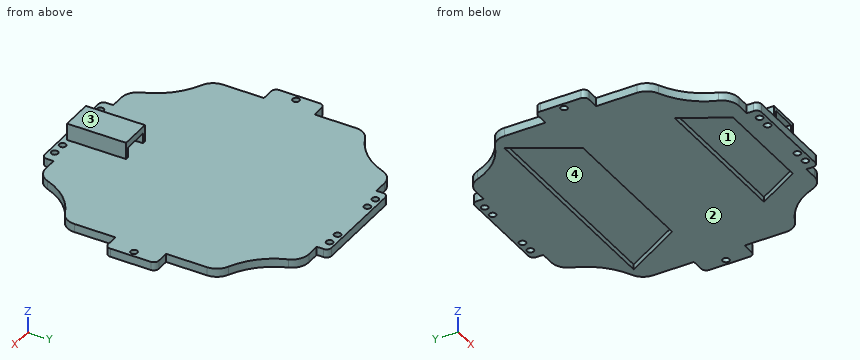
```python
from build123d import *

# Parameters (mm, degrees)
BOSS_EXTRUDE1_DEPTH = 5
SKETCH2_R           = 2
CUT_EXTRUDE1_DEPTH  = 5
CUT_EXTRUDE2_DEPTH  = 3
SKETCH4_W           = 19
SKETCH4_H           = 35
BOSS_EXTRUDE2_DEPTH = 10
SKETCH6_W           = 15
SKETCH6_H           = 8
CUT_EXTRUDE4_DEPTH  = 33
SKETCH7_W           = 15
SKETCH7_H           = 6
CUT_EXTRUDE5_DEPTH  = 2


with BuildPart() as part:
    # Sketch1 → Boss-Extrude1 (new body)
    with BuildSketch(Plane.XY):
        with BuildLine():
            Line((82, 15), (74.70882917, 15))
            Line((74.70882917, 15), (74.70882917, 39.302424721))
            ThreePointArc((74.70882917, 39.302424721), (73.092812163, 44.753005348), (68.767063336, 48.441939777))
            ThreePointArc((68.767063336, 48.441939777), (55.730177295, 57.736884279), (47.382982574, 71.4))
            ThreePointArc((47.382982574, 71.4), (43.723290865, 76.185352772), (37.978728218, 78))
            Line((37.978728218, 78), (30, 78))
            Line((30, 78), (30, 82))
            ThreePointArc((30, 82), (29.121320344, 84.121320344), (27, 85))
            Line((27, 85), (-27, 85))
            ThreePointArc((-27, 85), (-29.121320344, 84.121320344), (-30, 82))
            Line((-30, 82), (-30, 78))
            Line((-30, 78), (-37.978728218, 78))
            ThreePointArc((-37.978728218, 78), (-43.723290865, 76.185352772), (-47.382982574, 71.4))
            ThreePointArc((-47.382982574, 71.4), (-55.730177295, 57.736884279), (-68.767063336, 48.441939777))
            ThreePointArc((-68.767063336, 48.441939777), (-73.092812163, 44.753005348), (-74.70882917, 39.302424721))
            Line((-74.70882917, 39.302424721), (-74.70882917, 15))
            Line((-74.70882917, 15), (-82, 15))
            ThreePointArc((-82, 15), (-84.121320344, 14.121320344), (-85, 12))
            Line((-85, 12), (-85, -12))
            ThreePointArc((-85, -12), (-84.121320344, -14.121320344), (-82, -15))
            Line((-82, -15), (-74.70882917, -15))
            Line((-74.70882917, -15), (-74.70882917, -39.302424721))
            ThreePointArc((-74.70882917, -39.302424721), (-73.092812163, -44.753005348), (-68.767063336, -48.441939777))
            ThreePointArc((-68.767063336, -48.441939777), (-55.730177295, -57.736884279), (-47.382982574, -71.4))
            ThreePointArc((-47.382982574, -71.4), (-43.723290865, -76.185352772), (-37.978728218, -78))
            Line((-37.978728218, -78), (-30, -78))
            Line((-30, -78), (-30, -82))
            ThreePointArc((-30, -82), (-29.121320344, -84.121320344), (-27, -85))
            Line((-27, -85), (27, -85))
            ThreePointArc((27, -85), (29.121320344, -84.121320344), (30, -82))
            Line((30, -82), (30, -78))
            Line((30, -78), (37.978728218, -78))
            ThreePointArc((37.978728218, -78), (43.723290865, -76.185352772), (47.382982574, -71.4))
            ThreePointArc((47.382982574, -71.4), (55.730177295, -57.736884279), (68.767063336, -48.441939777))
            ThreePointArc((68.767063336, -48.441939777), (73.092812163, -44.753005348), (74.70882917, -39.302424721))
            Line((74.70882917, -39.302424721), (74.70882917, -15))
            Line((74.70882917, -15), (82, -15))
            ThreePointArc((82, -15), (84.121320344, -14.121320344), (85, -12))
            Line((85, -12), (85, 12))
            ThreePointArc((85, 12), (84.121320344, 14.121320344), (82, 15))
        make_face()
    extrude(amount=BOSS_EXTRUDE1_DEPTH)

    # Sketch2 → Cut-Extrude1 (cut)
    with BuildSketch(Plane(origin=(0, 0, 0), x_dir=(-1, 0, 0), z_dir=(0, 0, -1))):
        with Locations((81.5, 0)):
            Circle(SKETCH2_R)
        with Locations(Location((-81.5, 0, 0), (0, 0, 180))):
            Circle(SKETCH2_R)
        with Locations((-23, 81.5)):
            Circle(SKETCH2_R)
        with Locations((15, 81.5)):
            Circle(SKETCH2_R)
        with Locations((23, 81.5)):
            Circle(SKETCH2_R)
        with Locations((-15, 81.5)):
            Circle(SKETCH2_R)
        with Locations(Location((-23, -81.5, 0), (0, 0, 180))):
            Circle(SKETCH2_R)
        with Locations(Location((-15, -81.5, 0), (0, 0, 180))):
            Circle(SKETCH2_R)
        with Locations(Location((15, -81.5, 0), (0, 0, 180))):
            Circle(SKETCH2_R)
        with Locations(Location((23, -81.5, 0), (0, 0, 180))):
            Circle(SKETCH2_R)
    extrude(amount=-CUT_EXTRUDE1_DEPTH, mode=Mode.SUBTRACT)

    # Sketch3 → Cut-Extrude2 (cut)
    with BuildSketch(Plane(origin=(0, 0, 0), x_dir=(-1, 0, 0), z_dir=(0, 0, -1))):
        Polygon((-30, -70), (-45, -44.019237886), (45, -44.019237886), (30, -70), align=None)
        Polygon((65, 45), (-65, 45), (-45, 10.358983849), (45, 10.358983849), align=None)
    extrude(amount=-CUT_EXTRUDE2_DEPTH, mode=Mode.SUBTRACT)

    # Sketch4 → Boss-Extrude2 (add)
    with BuildSketch(Plane.XY.offset(5)):
        with Locations((0.2, -64.5)):
            Rectangle(SKETCH4_W, SKETCH4_H)
    extrude(amount=BOSS_EXTRUDE2_DEPTH)

    # Sketch6 → Cut-Extrude4 (cut)
    with BuildSketch(Plane.XZ.offset(82)):
        with Locations((0.2, 9)):
            Rectangle(SKETCH6_W, SKETCH6_H)
    extrude(amount=-CUT_EXTRUDE4_DEPTH, mode=Mode.SUBTRACT)

    # Sketch7 → Cut-Extrude5 (cut)
    with BuildSketch(Plane(origin=(0, -47, 0), x_dir=(1, 0, 0), z_dir=(0, 1, 0))):
        with Locations((0.2, -8)):
            Rectangle(SKETCH7_W, SKETCH7_H)
    extrude(amount=-CUT_EXTRUDE5_DEPTH, mode=Mode.SUBTRACT)


solid = part.part
```
Part model, mm, in its own coordinate system. Face numbers are marked on the shaded views. A direction names the side the tool comes from. Coordinates: 2 decimals unless noted, no trailing zeros. Write each loop counter-clockwise with the first axis right and the second up, starting at its lowest first coordinate (ties: lowest second). Pieces come first, ordered by that corner, then holes.
Item 1: Slice it at A-A (z = 8.75). Write the cut outline in (x, y), and give its area (3 significant figures).
Item 2: Which spindle directions (+Z, -Z, +X, -X, +Y, -Y) get a long thin tool onto all of the face, cutting with end or side? Do the marked faces 1 and 2. Say none if no direction does.
Item 3: Slice it at D-D (y = 36). Write the cut outline in (x, z), and give its area (3 significant figures).
Item 4: Slice it at C-C (x = 15). Write the cut outline in (y, z).
Item 5: Slice it at B-B (y = 0). Write the cut outline in (x, z), and give its area (3 significant figures).
Item 6: Probe line 1 (Y direction, x = -15, z = 3.2); line 2 (X direction, y = -81.5, z = 2.15); line 3 (Y direction, x = 23, z = 1.65). List the from-to ranges inside material, lowest first.
Item 7: Pin check, flat tips, straight feed: pin 1 (2.5 mm diameter, centred on x = 33, z = 1.5, fed in from +Y); pin 2 (1.5 mm diameter, centred on y = 44.5, z = 6.5, fed in from +X); pin 3 (4 mm diameter, centred on y = 27.5, z = 3, fed in from -X); pin 4 (2 mm diameter, centred on y = -80.5, z = 2.5, fed in from -X). Stop position of each tip, or through.
Item 8: Mould opens along X. For the marked faces 3 and 4 say: released by +X, released by -X, zero draft, split by the parting line, or undercut.
Results found:
1. outline: (-9.3, -82) - (-7.3, -82) - (-7.3, -47) - (-9.3, -47) - close; (7.7, -82) - (9.7, -82) - (9.7, -47) - (7.7, -47) - close
1. area: 140 mm2
2. face 1: -Z
2. face 2: -Z, +X, -X, +Y, -Y
3. outline: (-74.71, 0) - (-59.8, 0) - (-59.8, 3) - (59.8, 3) - (59.8, 0) - (74.71, 0) - (74.71, 5) - (-74.71, 5) - close
3. area: 388 mm2
4. outline: (-85, 0) - (-83.5, 0) - (-83.5, 5) - (-85, 5) - close; (-79.5, 0) - (-70, 0) - (-70, 3) - (-44.02, 3) - (-44.02, 0) - (10.36, 0) - (10.36, 3) - (45, 3) - (45, 0) - (79.5, 0) - (79.5, 5) - (-79.5, 5) - close; (83.5, 0) - (85, 0) - (85, 5) - (83.5, 5) - close
5. outline: (-85, 0) - (-83.5, 0) - (-83.5, 5) - (-85, 5) - close; (-79.5, 0) - (79.5, 0) - (79.5, 5) - (-79.5, 5) - close; (83.5, 0) - (85, 0) - (85, 5) - (83.5, 5) - close
5. area: 810 mm2
6. line 1: y = -85 to -83.5, -79.5 to 79.5, 83.5 to 85
6. line 2: x = -30 to -25, -21 to -17, -13 to 13, 17 to 21, 25 to 30
6. line 3: y = -85 to -83.5, -79.5 to -70, -44.02 to 10.36, 45 to 79.5, 83.5 to 85
7. pin 1: stops at y = 78
7. pin 2: passes through
7. pin 3: stops at x = -74.71
7. pin 4: stops at x = -30
8. face 3: zero draft
8. face 4: undercut
